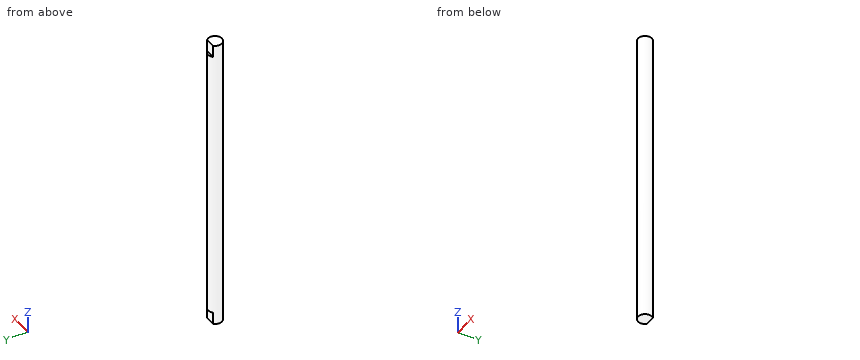
Autodesk Inventor part; units mm, degrees
ref_plane "YZ Plane" through (0, 0, 0) normal (1, 0, 0) x (0, 1, 0)
ref_plane "XZ Plane" through (0, 0, 0) normal (0, 1, 0) x (-1, 0, 0)
ref_plane "XY Plane" through (0, 0, 0) normal (0, 0, 1) x (1, 0, 0)
sketch "Sketch2" plane through (0, 0, 0) normal (0, 0, 1) x (1, 0, 0)
  circle A0 centre (0, 0) radius 8.5
  dimension "d4" = 17
extrude "Extrusion2" add sketch "Sketch2" along normal blind 370
sketch "Sketch3" plane through (0, 0, 370) normal (0, 0, 1) x (1, 0, 0)
  circle A0 centre (0, 0) radius 8.5
  arc A1 (6.0104, 6.0104) -> (-6.0104, 6.0104) centre (0, 0) ccw
  line L0 (0, 0) -> (6.0104, 6.0104) construction
  line L1 (0, 0) -> (8.5, 0) construction
  line L2 (0, 0) -> (-6.0104, 6.0104) construction
  arc A2 (6.0104, 6.0104) -> (-6.0104, 6.0104) centre (0, 0) ccw
  line L3 (6.0104, 6.0104) -> (-6.0104, 6.0104)
  point P0 (-6.0104, 6.0104)
  dimension "d7" = 45
extrude "Extrusion3" cut sketch "Sketch3" against normal blind 15 contours L3 A0 picked at (-0.3172, 6.8225)
sketch "Sketch4" plane through (0, 0, 0) normal (0, 0, -1) x (-1, 0, 0)
  arc A0 (-6.0104, 6.0104) -> (6.0104, 6.0104) centre (0, 0) ccw
  arc A1 (6.0104, 6.0104) -> (-6.0104, 6.0104) centre (0, 0) ccw
  line L0 (0, 0) -> (-6.0104, 6.0104) construction
  line L1 (0, 0) -> (6.0104, 6.0104) construction
  arc A2 (-6.0104, 6.0104) -> (6.0104, 6.0104) centre (0, 12.0208) ccw
  line L2 (-6.0104, 6.0104) -> (6.0104, 6.0104)
  line L3 (-6.0104, 6.0104) -> (6.0104, 6.0104)
  dimension "d11" = 90
extrude "Extrusion4" cut sketch "Sketch4" against normal blind 15 contours A1 L2
properties part number "Project_stationary_rod"
Verification items for the finished model (mm, model axes). Round coordinates to 2 decimals unless told otherwise and drop trailing zeros. Loops run counter-clockwise (first coordinate to the right, second up) from the corner with the lowest first, then second, coordinate; pieces in that order, holes last. Notation, with made-up numbers: (17, 41) - (64, 41) arc R34 ccw to (64, 72) - close; hole circle Ø9 at (-5, 16.5). An arc over 180 degrees is marked (long way). Use a Markdown table: item, result. Add a question column.
1. Section check B-B, the plane x = 3. Record the boundary of the cut face in (y, z).
2. Section check A-A, the plane z = 34. Record the boundary of the cut face in (x, y), plus the area to 3 significant figures.
3. Section check C-C, the plane y = -3.25. Record the boundary of the cut face in (x, z).
4. Gauge pin test, flat ends, axial feed: pin 1 (2 mm diameter, centred on x = 2.5, y = 8, fed in from +Z); pin 2 (3 mm diameter, centred on x = -6.5, z = 157, fed in from -Y); pin 3 (3.5 mm diameter, centred on x = 1.5, z = 363.5, fed in from +Y). Record the tip position at first contact, or that the pin passes through.
5. Thickness scan on probe 1 along X at (y, z) = (-0.5, 271.5); probe 2 along Z at (x, y) = (1.25, 8.25). Record the ranges inside material, lowest first. Write a range as [from, to].
Checks:
| question | item | result |
|---|---|---|
| 1 | outline | (-7.95, 0) - (6.01, 0) - (6.01, 15) - (7.95, 15) - (7.95, 355) - (6.01, 355) - (6.01, 370) - (-7.95, 370) - close |
| 2 | outline | circle Ø17 at (0, 0) |
| 2 | area | 227 mm^2 |
| 3 | outline | (-7.85, 0) - (7.85, 0) - (7.85, 370) - (-7.85, 370) - close |
| 4 | pin 1 | stops at z = 355 |
| 4 | pin 2 | stops at y = -6.87 |
| 4 | pin 3 | stops at y = 6.01 |
| 5 | probe 1 | x = [-8.49, 8.49] |
| 5 | probe 2 | z = [15, 355] |
